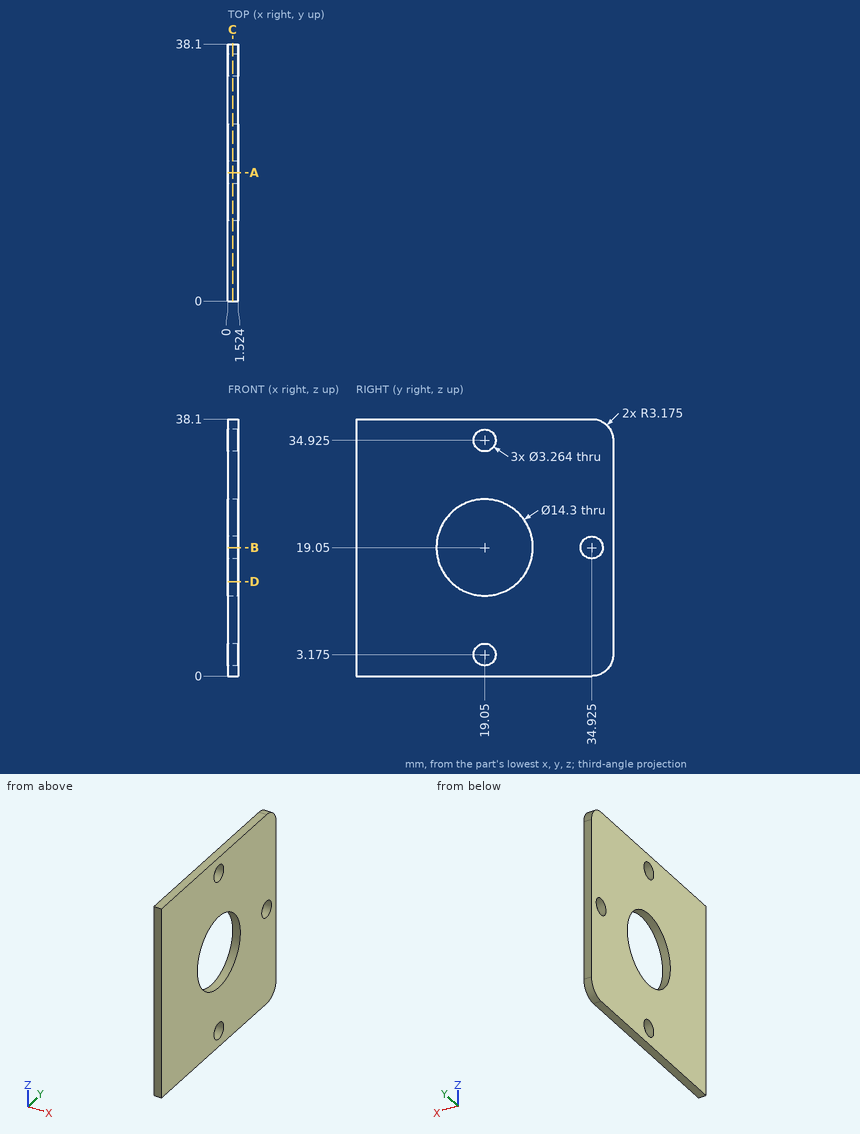
Part print with two shaded views. Sizes in mm from the minimum x, y, z corner. Coordinates: 2 decimals unless noted, no trailing zeros. Write each loop counter-clockwise with the first axis right and the second up, starting at its lowest first coordinate (ties: lowest second). Pieces come first, ordered by that corner, then holes. Notation, with made-up numbers: (-15.5, -8) - (-2.5, -8) arc R20 cw to (-2.5, -2) - close; hole circle Ø10 at (79.25, -21.75). An arc over 180 degrees is marked (long way). Use a Markdown table: item, result. Add a question column.
Item 1: Drop a flat-ended pin along its axis: pin 1 (4 mm diameter, centred on y = 19.05, z = 3.175, fed in from +X). Give the stop position or say it passes through.
Item 2: Band-saw the part on B-B, the plane z = 19.05. Write the cut outline in (x, y), and give its area (3 significant figures).
Item 3: Drill centre lines: line 1 along Y through (x, z) = (0.45, 19.05); line 2 along Y through (x, z) = (0.6, 3) (1 decimal); line 3 along Z through (x, y) = (1.25, 20). Where is each one in solid material? Low to high.
Item 4: Band-saw the part on A-A, the plane y = 19.05. Write the cut outline in (x, z), and give its area (3 significant figures).
Item 5: Band-saw the part on C-C, the plane x = 0.7. Give the number of separate pieces and of enclosed holes in the cut face, and give its area (3 significant figures).
Item 6: Band-saw the part on D-D, the plane z = 14. Write the cut outline in (x, y).
A:
| question | item | result |
|---|---|---|
| 1 | pin 1 | stops at x = 1.52 |
| 2 | outline | (0, 0) - (1.52, 0) - (1.52, 11.9) - (0, 11.9) - close; (0, 26.2) - (1.52, 26.2) - (1.52, 33.29) - (0, 33.29) - close; (0, 36.56) - (1.52, 36.56) - (1.52, 38.1) - (0, 38.1) - close |
| 2 | area | 31.3 mm² |
| 3 | line 1 | y = 0 to 11.9, 26.2 to 33.29, 36.56 to 38.1 |
| 3 | line 2 | y = 0 to 17.4, 20.7 to 38.1 |
| 3 | line 3 | z = 0 to 1.85, 4.5 to 11.96, 26.14 to 33.6, 36.25 to 38.1 |
| 4 | outline | (0, 0) - (1.52, 0) - (1.52, 1.54) - (0, 1.54) - close; (0, 4.81) - (1.52, 4.81) - (1.52, 11.9) - (0, 11.9) - close; (0, 26.2) - (1.52, 26.2) - (1.52, 33.29) - (0, 33.29) - close; (0, 36.56) - (1.52, 36.56) - (1.52, 38.1) - (0, 38.1) - close |
| 4 | area | 26.3 mm² |
| 5 | separate pieces | 1 |
| 5 | enclosed holes | 4 |
| 5 | area | 1,260 mm² |
| 6 | outline | (0, 0) - (1.52, 0) - (1.52, 13.99) - (0, 13.99) - close; (0, 24.11) - (1.52, 24.11) - (1.52, 38.1) - (0, 38.1) - close |
